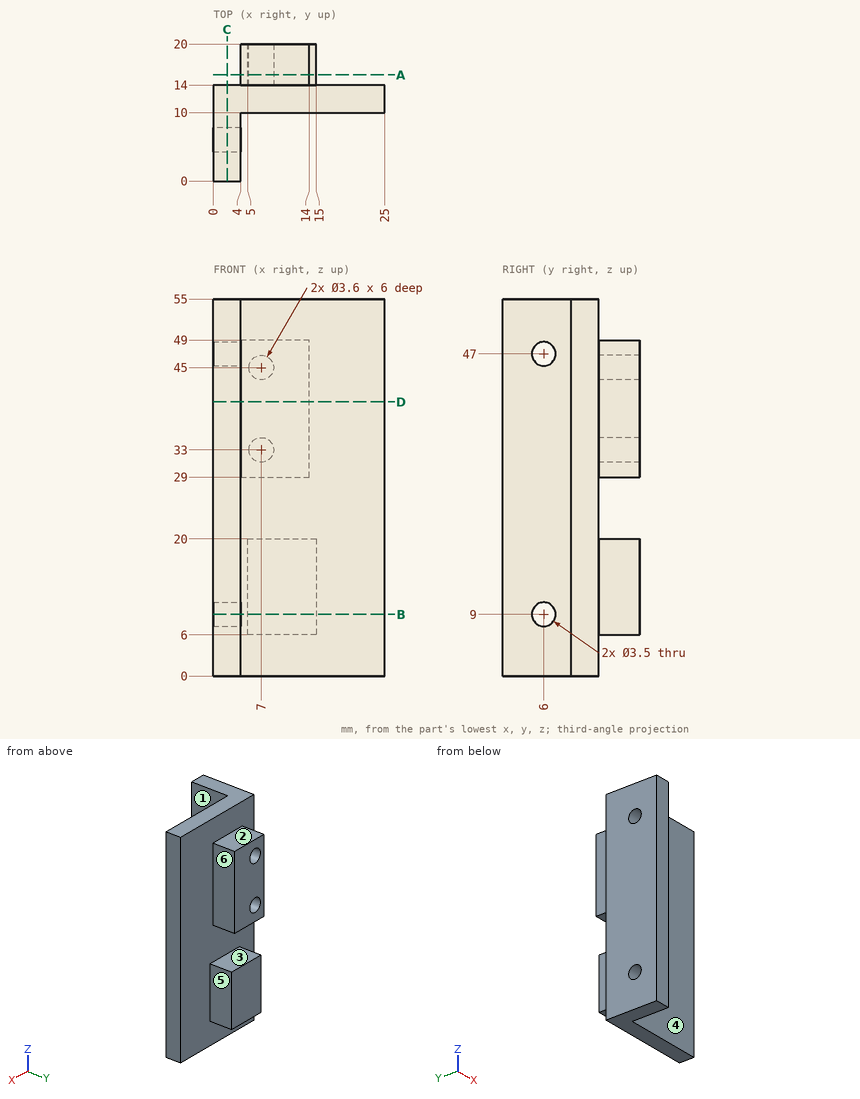
Here's the drawing with two shaded views (mm, measured from the low corner). I have some questions. A direction names the side the tool comes from. Give positions to 0.01 mm unless a question says otherwise; leave off trailing zeros. Order: outer loops, then holes, each group sorted by start corner. A loop starts at its lowest first (then second) coordinate and runs counter-clockwise, first axis right, second up. Notation, with made-up numbers: (56.5, -24) -> (72.5, -24) arc R26 ccw to (72.5, 2) -> close; hole circle Ø2 at (-16.75, 45.5). An arc over 180 degrees is marked (long way). One line per item, written item: value. Start each with the question number.
1. Will these pins go through, and if not, where does the flat tip stop? pin 1 Ø2 at (x, z) = (14.5, 36) entering from -Y; pin 2 Ø1.8 at (y, z) = (18, 13) entering from +X; pin 3 Ø1.8 at (x, z) = (6.5, 33) entering from +Y; pin 4 Ø3 at (y, z) = (6, 47) entering from -X.
2. We'd pull the mould along Z, two halves only. Please class the marked faces 1, 2 and 3: released by +Z, released by -Z, zero draft, split by the parting line, or undercut.
3. Imagine slicing it at D-D, the plane z = 40. List the corners of the cut face in (x, y) for me, plus the area to 3 significant figures.
4. I need wall thicknesses on probe 1 along Z at (x, y) = (7, 17); probe 2 along Z at (x, y) = (2.95, 6); probe 3 along Z at (x, y) = (9, 18.5). Which ranges of each line are inside material? Lowest first, please. Write a range as from..to.
5. For the marked faces 4, 5 and 6, which set-ups out of +Z, -Z, +X, -X, +Y, -Y let a thin tool reach every point of the face, with its end or its side?
6. Imagine slicing it at C-C, the plane x = 2. List the corners of the cut face in (y, z) for me, plus the area to 3 significant figures.
7. Imagine slicing it at B-B, the plane z = 9. List the corners of the cut face in (x, y) for me, plus the area to 3 significant figures.
8. Imagine slicing it at A-A, the plane y = 15.5. List the corners of the cut face in (x, z) for me.
Values follow:
1. pin 1: stops at y = 10
1. pin 2: stops at x = 15
1. pin 3: stops at y = 14
1. pin 4: passes through
2. face 1: zero draft
2. face 2: released by +Z
2. face 3: undercut
3. outline: (0, 0) -> (4, 0) -> (4, 10) -> (25, 10) -> (25, 14) -> (14, 14) -> (14, 20) -> (4, 20) -> (4, 14) -> (0, 14) -> close
3. area: 200 mm2
4. probe 1: z = 6..20, 29..31.2, 34.8..43.2, 46.8..49
4. probe 2: z = 0..7.25, 10.75..45.25, 48.75..55
4. probe 3: z = 6..20, 29..49
5. face 4: +Z, -Z, +X, -Y
5. face 5: +Z, -Z, +X, +Y
5. face 6: +Z, +X, +Y
6. outline: (0, 0) -> (14, 0) -> (14, 55) -> (0, 55) -> close; hole circle Ø3.5 at (6, 9); hole circle Ø3.5 at (6, 47)
6. area: 751 mm2
7. outline: (0, 0) -> (4, 0) -> (4, 4.25) -> (0, 4.25) -> close; (0, 7.75) -> (4, 7.75) -> (4, 10) -> (25, 10) -> (25, 14) -> (15, 14) -> (15, 20) -> (5, 20) -> (5, 14) -> (0, 14) -> close
7. area: 186 mm2
8. outline: (4, 29) -> (14, 29) -> (14, 49) -> (4, 49) -> close; (5, 6) -> (15, 6) -> (15, 20) -> (5, 20) -> close; hole circle Ø3.6 at (7, 33); hole circle Ø3.6 at (7, 45)
